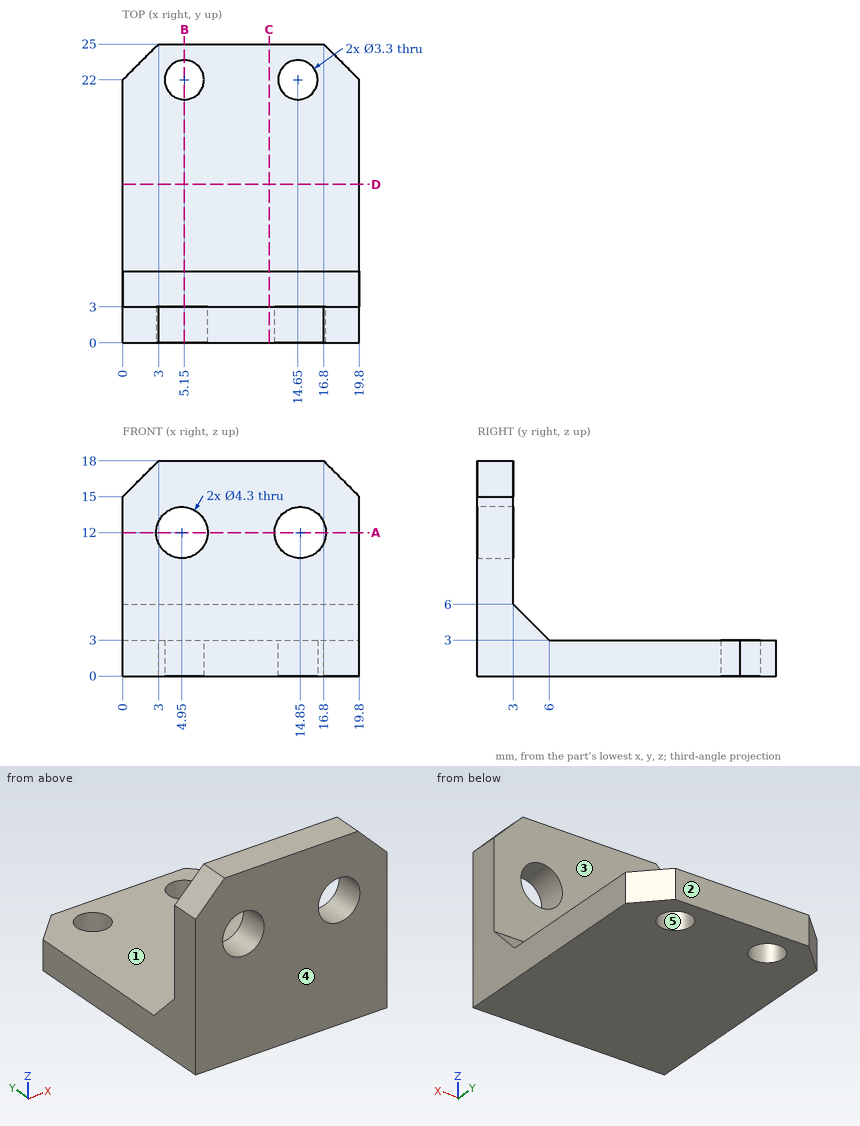
Here's the drawing with two shaded views (mm, measured from the low corner). I have some questions. A direction names the side the tool comes from. Round coordinates to 2 decimals unless told otherwise and drop trailing zeros. Order: outer loops, then holes, each group sorted by start corner. A loop starts at its lowest first (then second) coordinate and runs counter-clockwise, first axis right, second up. Notation, with made-up numbers: (68, -24.5) -> (97, -24.5) arc R21 ccw to (97, 3.5) -> close; hole circle Ø2 at (-23, 46.25). An arc over 180 degrees is marked (long way). Write each question's results on one line, items separated by ' | '. Start each with the question number.
Item 1: Will these pins go through, and if not, where does the flat tip stop? pin 1 (2.5 mm diameter, centred on x = 5.15, y = 22, fed in from -Z); pin 2 (9.5 mm diameter, centred on x = 6, z = 12.5, fed in from +Y).
Item 2: If we section it at A-A, the plane z = 12: Write out the boundary of the cut face in (x, y), then the cut area to 3 significant figures.
Item 3: If we section it at B-B, the plane x = 5.15: Write out the boundary of the cut face in (y, z).
Item 4: Thinking about a two-plate mould opening in Y: for the marked faces 3, 4 and 5, which applies, +Y half, -Y half, draft (parallel to the pull), parting line (faces both ways), or undercut?
Item 5: Which directions (+Z, -Z, +X, -X, +Y, -Y) give clear straight access to the entire face, cutting with the end or side of a thin tool? Please do the marked faces 1 and 2.
Item 6: If we section it at C-C, the plane x = 12.25: Write out the boundary of the cut face in (y, z).
Item 7: Please list where these lines run through material, in increasing order: L1, parallel to Y at x = 5.15, z = 0.7; L2, parallel to Y at x = 11, z = 7.
Item 8: If we section it at D-D, the plane y = 13.25: Write out the boundary of the cut face in (x, z).
Results:
1) pin 1: passes through | pin 2: stops at y = 3
2) outline: (0, 0) -> (2.8, 0) -> (2.8, 3) -> (0, 3) -> close; (7.1, 0) -> (12.7, 0) -> (12.7, 3) -> (7.1, 3) -> close; (17, 0) -> (19.8, 0) -> (19.8, 3) -> (17, 3) -> close | area: 33.6 mm2
3) outline: (0, 0) -> (20.35, 0) -> (20.35, 3) -> (6, 3) -> (3, 6) -> (3, 9.86) -> (0, 9.86) -> close; (0, 14.14) -> (3, 14.14) -> (3, 18) -> (0, 18) -> close; (23.65, 0) -> (25, 0) -> (25, 3) -> (23.65, 3) -> close
4) face 3: +Y half | face 4: -Y half | face 5: undercut
5) face 1: +Z, +X, -X, +Y | face 2: +Z, -Z, +X, -X, +Y
6) outline: (0, 0) -> (25, 0) -> (25, 3) -> (6, 3) -> (3, 6) -> (3, 18) -> (0, 18) -> close
7) L1: y = 0 to 20.35, 23.65 to 25 | L2: y = 0 to 3
8) outline: (0, 0) -> (19.8, 0) -> (19.8, 3) -> (0, 3) -> close
